Can you work these out from the model? Positions are in its coordinate system, mm. Face numbers are marked on the shaded views. A direction names the side the tool comes from. Round coordinates to 2 decimals unless told otherwise and drop trailing zeros. Order: outer loops, then holes, each group sorted by start corner. A loop starts at its lowest first (then second) coordinate and runs counter-clockwise, first axis right, second up. Notation, with made-up numbers: (58.5, 6.25) -> (104.5, 6.25) arc R13 cw to (104.5, 17.25) -> close; hole circle Ø6 at (-35.5, -29.75). An arc over 180 degrees is marked (long way). Use a Markdown table: item, result. Add a question column.
Q1. If we section it at B-B on x = 82.5: List the corners of the cut face in (y, z) for me.
Q2. For the marked faces 1 and 2, which set-ups out of +Z, -Z, +X, -X, +Y, -Y let a thin tool reach every point of the face, with its end or its side?
Q3. I need wall thicknesses on line 1 along Z through (x, y) = (36, 28.5); line 2 along Z through (x, y) = (104, 30); line 3 along Z through (x, y) = (-81, 10). Which ranges of each line are inside material? Lowest first, please. Write a range as [from, to].
Q4. I'm going to push flat-ended pins straight in: pin 1 Ø1.5 at (x, z) = (97, -13.5) entering from -Y; pin 2 Ø6.5 at (y, z) = (29, 60.5) entering from -X; pin 3 Ø9.5 at (x, y) = (-74, 11) entering from -Z; pin 4 Ø10.5 at (x, z) = (-79.5, 43.5) entering from +Y. Where does each tip first touch, or does it pass through?
Q5. If we section it at C-C on z = -27: List the corners of the cut face in (x, y) for me.
Q6. We'd pull the mould along Z, two halves only. Please class the marked faces 3, 4 and 5: +Z half, -Z half, draft (parallel to the pull), parting line (faces both ways), or undercut.
Q7. If we section it at A-A on y = 23.5: List the corners of the cut face in (x, z) for me.
Q8. If we section it at D-D on z = 56: List the corners of the cut face in (x, y) for me, plus the area to 3 significant figures.
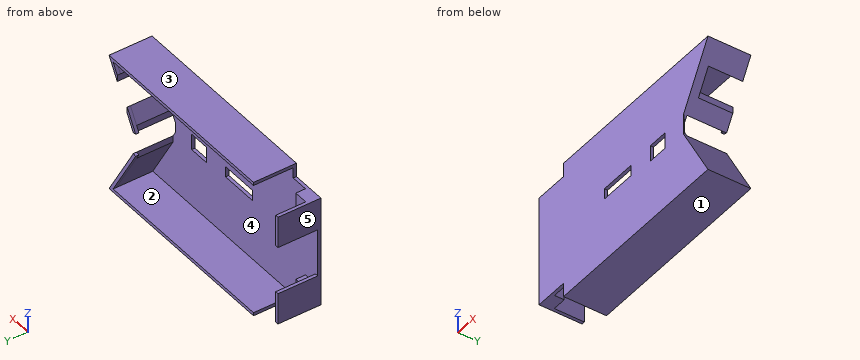
```python
from build123d import *

# Parameters (mm, degrees)
BOSS_EXTRUDE1_DEPTH = 40
SHELL5_START        = 3
SHELL5_DEPTH        = 34
CHAMFER1_SIZE       = 3
CUT_EXTRUDE1_DEPTH  = 3
SKETCH7_W           = 13
SKETCH7_H           = 9
CUT_EXTRUDE3_DEPTH  = 10
SKETCH7_4_W         = 13
SKETCH7_4_H         = 9
BOSS_EXTRUDE7_DEPTH = 30
CUT_EXTRUDE8_DEPTH  = 55
SKETCH7_6_W         = 13
SKETCH7_6_H         = 9
CUT_EXTRUDE10_DEPTH = 10
SKETCH8_W           = 45
SKETCH8_H           = 40
CUT_EXTRUDE4_DEPTH  = 30
SKETCH9_W           = 19.285714286
SKETCH9_H           = 15
SKETCH9_W_2         = 35
SKETCH9_H_2         = 10
CUT_EXTRUDE5_DEPTH  = 30


# Read off the part's stored shape, not the designer's step: Shell5
with BuildPart() as part:
    # Sketch1 → Boss-Extrude1 (new body)
    with BuildSketch(Plane(origin=(0, 0, 0), x_dir=(1, 0, 0), z_dir=(0, 1, 0))):
        Polygon((-90, -65), (130.754264805, -65), (99, -10), (99, 10), (130.754264805, 65), (-90, 65), align=None)
    extrude(amount=BOSS_EXTRUDE1_DEPTH)

    # Shell5 outline → Shell5 (cut)
    with BuildSketch(Plane(origin=(0, 0, 0), x_dir=(1, 0, 0), z_dir=(0, 1, 0)).offset(SHELL5_START)):
        Polygon((99, -16), (99, 16), (125.558112383, 62), (-87, 62), (-87, -62), (125.558112383, -62), align=None)
    extrude(amount=SHELL5_DEPTH, mode=Mode.SUBTRACT)

    # Chamfer1
    chamfer1_edges = [part.edges().sort_by_distance(p)[0] for p in [
        (99, 3, 0),
    ]]
    chamfer(chamfer1_edges, length=CHAMFER1_SIZE - 0.0001)  # a hair under: the kernel refuses the full size

    # Sketch6 → Cut-Extrude1 (cut)
    with BuildSketch(Plane(origin=(0, 40, 0), x_dir=(1, 0, 0), z_dir=(0, 1, 0))):
        Polygon((125.558112383, 62), (-87, 62), (-87, -62), (125.558112383, -62), (96, -10.803847577), (96, 10.803847577), align=None)
        Polygon((99, 10), (96, 10.803847577), (96, -10.803847577), (99, -10), align=None)
    extrude(amount=-CUT_EXTRUDE1_DEPTH, mode=Mode.SUBTRACT)

    # Sketch7 → Cut-Extrude3 (cut)
    with BuildSketch(Plane(origin=(0, 0, 62), x_dir=(-1, 0, 0), z_dir=(0, 0, -1))):
        Polygon((58, 3), (58, -4.5), (103, -4.5), (103, 40.5), (58, 40.5), (58, 40), (87, 40), (87, 12), (87, 3), (74, 3), align=None)
        Polygon((58, 40), (58, 3), (74, 3), (74, 12), (87, 12), (87, 40), align=None)
        with Locations((80.5, 7.5)):
            Rectangle(SKETCH7_W, SKETCH7_H)
    cut_extrude3 = extrude(amount=-CUT_EXTRUDE3_DEPTH, mode=Mode.SUBTRACT)

    # Sketch7<4> → Boss-Extrude7 (add)
    with BuildSketch(Plane(origin=(0, 0, 62), x_dir=(-1, 0, 0), z_dir=(0, 0, -1))):
        with Locations((80.5, 7.5)):
            Rectangle(SKETCH7_4_W, SKETCH7_4_H)
    boss_extrude7 = extrude(amount=BOSS_EXTRUDE7_DEPTH)

    # Sketch12 → Cut-Extrude8 (cut)
    with BuildSketch(Plane(origin=(0, 0, 62), x_dir=(-1, 0, 0), z_dir=(0, 0, -1))):
        Polygon((-107.058112383, 43), (-107.058112383, 8), (-120.058112383, 43), align=None)
        Polygon((-120.058112383, 43), (-120.058112383, 8), (-107.058112383, 8), align=None)
        Polygon((-107.058112383, 40), (-118.943826668, 40), (-107.058112383, 8), align=None)
    extrude(amount=CUT_EXTRUDE8_DEPTH, mode=Mode.SUBTRACT)

    # Sketch7<6> → Cut-Extrude10 (cut)
    with BuildSketch(Plane(origin=(0, 0, 62), x_dir=(-1, 0, 0), z_dir=(0, 0, -1))):
        Polygon((58, 3), (58, -4.5), (103, -4.5), (103, 40.5), (58, 40.5), (58, 40), (87, 40), (87, 12), (87, 3), (74, 3), align=None)
        with Locations((80.5, 7.5)):
            Rectangle(SKETCH7_6_W, SKETCH7_6_H)
        Polygon((58, 40), (58, 3), (74, 3), (74, 12), (87, 12), (87, 40), align=None)
    cut_extrude10 = extrude(amount=CUT_EXTRUDE10_DEPTH, mode=Mode.SUBTRACT)

    # Mirror6: Cut-Extrude3, Boss-Extrude7, Cut-Extrude10 across plane
    add(cut_extrude3.mirror(Plane.XY), mode=Mode.SUBTRACT)
    add(boss_extrude7.mirror(Plane.XY))
    add(cut_extrude10.mirror(Plane.XY), mode=Mode.SUBTRACT)

    # Sketch8 → Cut-Extrude4 (cut)
    with BuildSketch(Plane(origin=(-87, 0, 0), x_dir=(0, 0, -1), z_dir=(1, 0, 0))):
        with Locations((0, 23)):
            Rectangle(SKETCH8_W, SKETCH8_H)
    extrude(amount=-CUT_EXTRUDE4_DEPTH, mode=Mode.SUBTRACT)

    # Sketch9 → Cut-Extrude5 (cut)
    with BuildSketch(Plane(origin=(0, 3, 0), x_dir=(1, 0, 0), z_dir=(0, 1, 0))):
        with Locations((65, 0)):
            Rectangle(SKETCH9_W, SKETCH9_H)
        with Locations((12.857142857, 0)):
            Rectangle(SKETCH9_W_2, SKETCH9_H_2)
    extrude(amount=-CUT_EXTRUDE5_DEPTH, mode=Mode.SUBTRACT)


solid = part.part
```
Answer below:
| question | item | result |
|---|---|---|
| 1 | outline | (0, -65) -> (40, -65) -> (40, -62) -> (3, -62) -> (3, 62) -> (40, 62) -> (40, 65) -> (0, 65) -> close |
| 2 | face 1 | -Z, +X, -X, +Y, -Y |
| 2 | face 2 | -X, +Y |
| 3 | line 1 | [-65, -62], [62, 65] |
| 3 | line 2 | [-65, -62], [-24.66, -18.66], [18.66, 24.66], [62, 65] |
| 3 | line 3 | [-52, -32], [32, 52] |
| 4 | pin 1 | y = 0 |
| 4 | pin 2 | x = -58 |
| 4 | pin 3 | z = -52 |
| 4 | pin 4 | y = 12 |
| 5 | outline | (-90, 0) -> (108.81, 0) -> (108.81, 40) -> (105.35, 40) -> (105.35, 3) -> (-87, 3) -> (-87, 40) -> (-90, 40) -> close |
| 6 | face 3 | +Z half |
| 6 | face 4 | undercut |
| 6 | face 5 | draft |
| 7 | outline | (-90, -52) -> (-87, -52) -> (-87, -22.5) -> (-90, -22.5) -> close; (-90, 22.5) -> (-87, 22.5) -> (-87, 52) -> (-90, 52) -> close; (-58, -65) -> (130.75, -65) -> (99, -10) -> (99, -16) -> (125.56, -62) -> (-58, -62) -> close; (-58, 62) -> (125.56, 62) -> (120.06, 52.47) -> (120.06, 46.47) -> (130.75, 65) -> (-58, 65) -> close; (99, 10) -> (107.06, 23.96) -> (107.06, 29.96) -> (99, 16) -> close |
| 8 | outline | (-58, 0) -> (125.56, 0) -> (125.56, 40) -> (122.09, 40) -> (122.09, 3) -> (-58, 3) -> close |
| 8 | area | 679 mm² |
